Autodesk Inventor part; units mm, degrees
ref_plane "YZ Plane" through (0, 0, 0) normal (1, 0, 0) x (0, 1, 0)
ref_plane "XZ Plane" through (0, 0, 0) normal (0, 1, 0) x (-1, 0, 0)
ref_plane "XY Plane" through (0, 0, 0) normal (0, 0, 1) x (1, 0, 0)
sketch "Sketch1" plane through (0, 0, 0) normal (1, 0, 0) x (0, 1, 0)
  line L0 (6.35, -12.9887) -> (279.4, -12.9887)
  line L1 (279.4, -12.9887) -> (279.4, -19.3387)
  line L2 (279.4, -19.3387) -> (0, -19.3387)
  line L3 (0, -19.3387) -> (0, -12.9887)
  line L4 (0, -12.9887) -> (0, 114.0113)
  line L5 (0, 114.0113) -> (6.35, 114.0113)
  line L6 (6.35, 114.0113) -> (6.35, -12.9887)
  point P0 (0, 0)
  dimension "d0" = 279.4
  dimension "d1" = 6.35
  dimension "d2" = 127
  dimension "d3" = 6.35
extrude "Extrusion1" add sketch "Sketch1" against normal blind 19.05
sketch "Sketch2" plane through (0, 6.35, 114.0113) normal (0, 1, 0) x (1, 0, 0)
  line L0 (0, 127) -> (-19.05, 127)
  line L1 (-19.05, 127) -> (0, 127)
  line L2 (0, 0) -> (0, 133.35)
  point P0 (0, 114.0113)
fillet "Fillet1" radius 6.35 1 edges at (-9.525, 0, -19.3387)
bend part "Bend Part1" radius 6.35 angle 65 line through (-19.05, 6.35, -12.9887) along (1, 0, 0) centre toward (0, 1, 0) moving side (0, 0, 1) both sides no
sketch "Sketch3" plane through (0, 6.35, -19.3387) normal (0, 0, -1) x (-1, 0, 0)
  line L0 (39.6982, 130.9983) -> (-135.4768, 130.9983)
  line L1 (19.05, 118.2983) -> (0, 118.2983)
  point P0 (0, -6.35)
bend part "Bend Part2" radius 6.35 angle 45 line through (-19.05, 124.6483, -19.3387) along (1, 0, 0) centre toward (0, 0, -1) moving side (0, -1, 0) both sides no
properties part number "Plexi hooks"
Design review of the part built by this model. Coordinates are the model's own, in mm. A direction names the side the tool comes from. Round coordinates to 2 decimals unless told otherwise and drop trailing zeros. Loops run counter-clockwise (first coordinate to the right, second up) from the corner with the lowest first, then second, coordinate; pieces in that order, holes last. Notation, with made-up numbers: (57.25, 17.25) - (116.25, 17.25) arc R24 cw to (116.25, 38.25) - close; hole circle Ø5 at (32, -2). An arc over 180 degrees is marked (long way). One line per item, written item: value. Start each with the question number.
1) Consider section D-D on y = 186.5. Give the boundary of the cut face in (x, z).
2) Consider section C-C on x = -9.5. Give the boundary of the cut face in (y, z), then the cut area to 3 significant figures.
3) Consider section A-A on z = -56.5. Give the boundary of the cut face in (x, y).
4) For faces 1 (the flat face through (-9, 203, -19.339)), 2 (the flat face through (-9.392, 75.046, -57.331)), 3 (the cylindrical face through (-9.658, 119.724, -13.982)), list the 3-axis set-ups (+Z, -Z, +X, -X, +Y, -Y) from which the entire face can be reached by the end or side of a thin tool; tool diameter is ignored.
5) Consider section B-B on y = 65. Give the boundary of the cut face in (x, z).
6) Insertion check: pin 1 Ø5.5 at (x, y) = (-8.5, 208) entering from +Z; pin 2 Ø5.5 at (x, y) = (-7, 230) entering from -Z; pin 3 Ø3 at (x, y) = (-17, 89) entering from +Z. Each pin has a flat end and moves straight along its axis. Give the tip position at first contact, or say it passes through.
7) Draft analysis for pull direction Z (two halves, no side actions). For faces 4 (the cylindrical face through (-9.658, 33.847, -93.765)), 5 (the flat face through (-9, 279.4, -16)), 6 (the flat face through (-9, 201, -12.989)), state which applies: +Z half, -Z half, draft (parallel to the pull), parting line (faces both ways), or undercut.
8) To check wall thickness, follow L1, parallel to Z at x = -6.25, y = 191; L2, parallel to Y at x = -2.5, z = -57; L3, parallel to Y at x = -17, z = -75.5. State the ranges of each line that lie inside material, in increasing order. Write a range as from..to.
Reported:
1. outline: (-19.05, -19.34) - (0, -19.34) - (0, -12.99) - (-19.05, -12.99) - close
2. outline: (28.1, -88) arc R12.7 ccw to (31.05, -101.32) arc R6.35 ccw to (40.04, -101.32) - (120.16, -21.2) arc R6.35 cw to (124.65, -19.34) - (279.4, -19.34) - (279.4, -12.99) - (124.65, -12.99) arc R12.7 ccw to (115.67, -16.71) - (35.55, -96.83) arc R6.35 cw to (34.07, -90.17) - (75.04, 22.4) - (69.07, 24.57) - close
2. area: 2,610 mm^2
3. outline: (-19.05, 39.57) - (0, 39.57) - (0, 46.32) - (-19.05, 46.32) - close; (-19.05, 75.88) - (0, 75.88) - (0, 84.86) - (-19.05, 84.86) - close
4. face 1: -Z, +X, -X, +Y
4. face 2: +X, -X
4. face 3: +Z, +X, -X
5. outline: (-19.05, -76.36) - (0, -76.36) - (0, -67.38) - (-19.05, -67.38) - close; (-19.05, -5.18) - (0, -5.18) - (0, 13.38) - (-19.05, 13.38) - close
6. pin 1: stops at z = -12.99
6. pin 2: stops at z = -19.34
6. pin 3: stops at z = -41.88
7. face 4: undercut
7. face 5: draft
7. face 6: +Z half
8. L1: z = -19.34..-12.99
8. L2: y = 39.38..46.14, 75.38..84.36
8. L3: y = 32.65..39.41, 56.88..65.86
